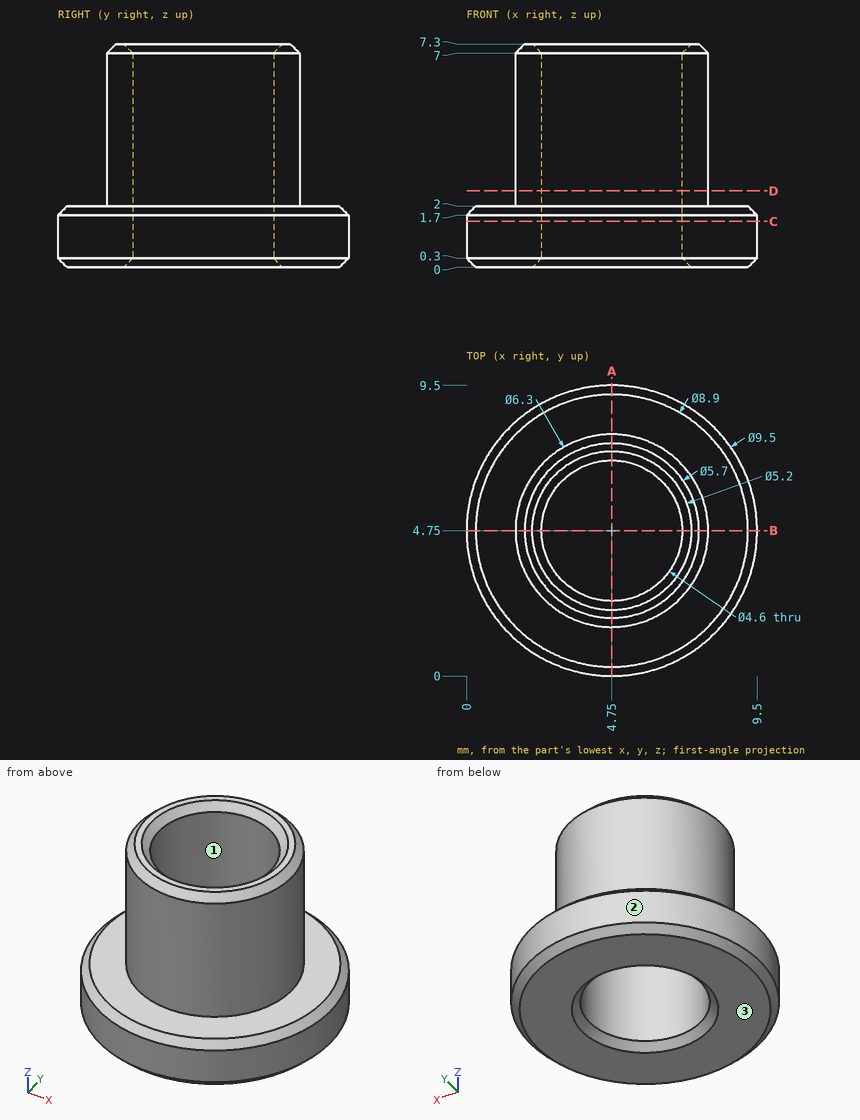
Geometry check sheet. Reference: drawing and pictorial views, mm from the part's lowest x, y, z. Give positions to 0.01 mm unless a question says otherwise; leave off trailing zeros. Loops run counter-clockwise (first coordinate to the right, second up) from the corner with the lowest first, then second, coordinate; pieces in that order, holes last. Notation, with made-up numbers: (-40, 75.25) - (-6, 75.25) arc R35 ccw to (-6, 112.25) - close; hole circle Ø9 at (68, 21.5). An arc over 180 degrees is marked (long way). One line per question, with ' | ' between items. Start each with the question number.
1. Material ranges on line 1 along Y through (x, z) = (4.75, 4.25); line 2 along Y through (x, z) = (4.75, 1); line 3 along Z through (x, y) = (1.5, 7.25), recorded low to high. Write a range as [from, to].
2. Cross-section at A-A, the plane x = 4.75. Enter the section's corners in (y, z), plus the area to 3 significant figures.
3. Cross-section at C-C, the plane z = 1.5. Enter the section's corners in (x, y).
4. Gauge pin test, flat ends, axial feed: pin 1 Ø4 at (x, y) = (4.75, 4.75) entering from -Z; pin 2 Ø3 at (x, z) = (3, 5.5) entering from +Y; pin 3 Ø4 at (y, z) = (8, 6) entering from -X. Record the tip position at first contact, or that the pin passes through.
5. Cross-section at D-D, the plane z = 2.5. Enter the section's corners in (x, y), plus the area to 3 significant figures.
6. Draft check along Y on the marked faces 1, 2 and 3. Enter one of: released by +Y, released by -Y, zero draft, split by the parting line, or undercut.
Check result:
1) line 1: y = [1.6, 2.45], [7.05, 7.9] | line 2: y = [0, 2.45], [7.05, 9.5] | line 3: z = [0, 2]
2) outline: (0, 0.3) - (0.3, 0) - (2.15, 0) - (2.45, 0.3) - (2.45, 7) - (2.15, 7.3) - (1.9, 7.3) - (1.6, 7) - (1.6, 2) - (0.3, 2) - (0, 1.7) - close; (7.05, 0.3) - (7.35, 0) - (9.2, 0) - (9.5, 0.3) - (9.5, 1.7) - (9.2, 2) - (7.9, 2) - (7.9, 7) - (7.6, 7.3) - (7.35, 7.3) - (7.05, 7) - close | area: 18.4 mm2
3) outline: circle Ø9.5 at (4.75, 4.75); hole circle Ø4.6 at (4.75, 4.75)
4) pin 1: passes through | pin 2: stops at y = 7.89 | pin 3: stops at x = 1.86
5) outline: circle Ø6.3 at (4.75, 4.75); hole circle Ø4.6 at (4.75, 4.75) | area: 14.6 mm2
6) face 1: undercut | face 2: split by the parting line | face 3: zero draft
